The listing builds one solid part. Answer for the finished solid, in the listing's coordinates (mm). A direction names the side the tool comes from. Give positions to 0.01 mm unless a question says otherwise; leave off trailing zeros. Write each loop counter-clockwise with the first axis right and the second up, starting at its lowest first coordinate (ties: lowest second). Pieces come first, ordered by that corner, then holes. Notation, with made-up numbers: (23, 64) - (60, 64) arc R33 ccw to (60, 95) - close; hole circle Ø3 at (59.5, 39). An arc over 180 degrees is marked (long way). Write each question's results on one line, items separated by ' | '. Start each with the question number.
Q1. Section B-B (x = 0) is taken. State how many separate pieces and enclosed holes the cut face has, plus the area to 3 significant figures.
Q2. For faces 4 (the face through (0.364, 0.967, 18.076)), 5 (the face through (-0.28, 10.312, 33.866)), 6 (the face through (-10.325, -1.464, 1.479)), 7 (the face through (0, 13, 2)), 8 (the face through (0, 3, 4)), determine the directions among +Z, -Z, +X, -X, +Y, -Y from which every point of the face is accessible in a straight line to the end or side of a thin tool.
Q3. Section A-A (z = 8) is taken. Determine the outline of the cut face in (x, y), plus the area to 3 significant figures.
Q4. Section C-C (y = 41.5) is taken. Determine the outline of the cut face in (x, z).
Q5. For a pull along Z with two mould halves and no side action, classify faces 1 (the face through (-18.498, 44.726, 45.771)), 2 (the face through (-9.3, 1.5, 3)), 3 (the face through (-28, 14.7, 15.4)) as pulls with the +Z half, pulls with the -Z half, needs draft (parallel to the pull), parting line crosses it, or undercut.
Q6. Find the intervals of material crossed by probe 1 along X at (y, z) = (0.5, 18); probe 2 along Z at (x, y) = (19.5, 25.5); probe 3 along Z at (x, y) = (0.5, 10.5), in increasing order.
Q7. Flat-ended cylindrical pins translate along their axes: pin 1 Ø6 at (x, z) = (-21.5, 15.5) entering from -Y; pin 2 Ø15 at (x, y) = (4, 30) entering from -Z; pin 3 Ø5 at (y, z) = (38.5, 42.5) entering from -X; pin 4 Ø4 at (x, z) = (-19, 15.5) entering from -Y. Find the tip coordinate at first contact, or state that the pin passes through.
```python
from build123d import *

# Parameters (mm, degrees)
SKETCH_1_R          = 1.4999999999999987
EXTRUDE_1_DEPTH     = 4
SKETCH_3_R          = 3.2499999999999996
SKETCH_3_R_2        = 3.249999999999999
CUT_EXTRUDE_1_DEPTH = 1
EXTRUDE_2_DEPTH     = 4
EXTRUDE_3_DEPTH     = 4
EXTRUDE_4_DEPTH     = 52
FILLET_1_R          = 25
FILLET_2_R          = 20
EXTRUDE_6_DEPTH     = 52
FILLET_4_R          = 6
FILLET_5_R          = 2
SKETCH_11_R         = 7.500000000000031
CUT_EXTRUDE_2_DEPTH = 4
FILLET_6_R          = 2


with BuildPart() as part:
    # 草图1 → 凸台-拉伸1 (new body)
    # profile 1 of 3: a face of its own
    with BuildSketch(Plane.XY):
        Polygon((30.00000000000006, 4.99999999999999), (30.000000000000057, -5.0000000000000115), (-29.99999999999994, -5.0000000000000115), (-29.999999999999936, 4.99999999999999), align=None)
        with Locations((9.999999999999996, 5.68e-15)):
            Circle(SKETCH_1_R, mode=Mode.SUBTRACT)
        with Locations((-10.000000000000004, -4.4e-16)):
            Circle(SKETCH_1_R, mode=Mode.SUBTRACT)
    # profile 2 of 3: a face of its own
    with BuildSketch(Plane.XY):
        Polygon((-30.000000000000014, 12.999999999999998), (29.999999999999986, 12.999999999999998), (30.00000000000006, 4.99999999999999), (-29.999999999999936, 4.99999999999999), align=None)
    # profile 3 of 3: a face of its own
    with BuildSketch(Plane.XY):
        Polygon((-29.99999999999994, -5.0000000000000115), (-30.000000000000018, -8.000000000000002), (29.999999999999982, -8.000000000000002), (30.000000000000057, -5.0000000000000115), align=None)
    extrude(amount=EXTRUDE_1_DEPTH)

    # 草图3 → 切除-拉伸1 (cut)
    with BuildSketch(Plane.XY.offset(4)):
        with Locations((-10.000000000000004, -4.6e-16)):
            Circle(SKETCH_3_R)
        with Locations((9.999999999999996, 5.69e-15)):
            Circle(SKETCH_3_R_2)
    extrude(amount=-CUT_EXTRUDE_1_DEPTH, mode=Mode.SUBTRACT)

    # 草图5 → 凸台-拉伸2 (add)
    with BuildSketch(Plane.ZY.offset(29.999999999999936)):
        Polygon((47.25000000000001, 15.99999999999999), (4, -8.000000000000012), (4, 12.999999999999988), (44.25, 18.99999999999999), (44.25, 64.99999999999999), (47.25, 64.99999999999999), align=None)
    extrude(amount=-EXTRUDE_2_DEPTH)

    # 草图6 → 凸台-拉伸3 (add)
    with BuildSketch(Plane(origin=(30.00000000000006, -1.041e-14, 0), x_dir=(0, 0, -1), z_dir=(1, -3.5e-16, 0))):
        Polygon((-44.25, 64.99999999999999), (-47.25, 64.99999999999999), (-47.25000000000001, 15.99999999999999), (-4, -8.00000000000001), (-4, 13.000000000000009), (-44.25, 18.999999999999993), align=None)
    extrude(amount=-EXTRUDE_3_DEPTH)

    # 草图7 → 凸台-拉伸4 (add)
    with BuildSketch(Plane(origin=(-25.999999999999932, 8.47e-15, 0), x_dir=(0, 0, -1), z_dir=(1, -3.3e-16, 0))):
        Polygon((-44.25, 14.335260115606923), (-44.25, 18.999999999999993), (-44.25, 64.99999999999999), (-47.25, 64.99999999999999), (-47.25000000000001, 15.999999999999986), align=None)
    extrude(amount=EXTRUDE_4_DEPTH)

    # 圆角1
    fillet_1_edges = [part.edges().sort_by_distance(p)[0] for p in [
        (-29.999999999999915, 65, 45.75),
        (30.00000000000008, 64.99999999999997, 45.75),
    ]]
    fillet(fillet_1_edges, radius=FILLET_1_R)

    # 圆角2
    fillet_2_edges = [part.edges().sort_by_distance(p)[0] for p in [
        (-27.99999999999993, 19, 44.25),
        (28.000000000000068, 18.999999999999982, 44.25),
    ]]
    fillet(fillet_2_edges, radius=FILLET_2_R)

    # 草图9 → 凸台-拉伸6 (add)
    with BuildSketch(Plane(origin=(-25.999999999999932, 8.47e-15, 0), x_dir=(0, 0, -1), z_dir=(1, -3.3e-16, 0))):
        Polygon((-33.14820415728187, 11.605667405253392), (-34.60384535674384, 8.982480660389633), (-17.11593372431879, -0.7217940026901655), (-17.115933724318786, 2.7091473962102923), align=None)
    extrude(amount=EXTRUDE_6_DEPTH)

    # 圆角4
    fillet_4_edges = [part.edges().sort_by_distance(p)[0] for p in [
        (-25.99999999999993, 10.294074032821522, 33.87602475701286),
        (26.00000000000007, 10.294074032821504, 33.87602475701286),
    ]]
    fillet(fillet_4_edges, radius=FILLET_4_R)

    # 圆角5
    fillet_5_edges = [part.edges().sort_by_distance(p)[0] for p in [
        (6.75e-14, -0.721794002690165, 17.11593372431879),
    ]]
    fillet(fillet_5_edges, radius=FILLET_5_R)

    # 草图11 → 切除-拉伸2 (cut)
    with BuildSketch(Plane.XY.offset(47.25000000000001)):
        with BuildLine():
            ThreePointArc((-20.11504932930021, 46.93210856983418), (-19.24913556906646, 44.8416078260319), (-17.158634825264187, 45.70752158626565))
            ThreePointArc((-17.158634825264187, 45.70752158626565), (-18.024548585497932, 47.79802233006792), (-20.11504932930021, 46.93210856983418))
        make_face()
        with BuildLine():
            ThreePointArc((-4.207521586267032, 24.341365174733916), (-6.298022330069304, 23.475451414500167), (-5.432108569835557, 21.384950670697894))
            ThreePointArc((-5.432108569835557, 21.384950670697894), (-3.341607826033282, 22.250864430931642), (-4.207521586267032, 24.341365174733916))
        make_face()
        with BuildLine():
            ThreePointArc((20.11504932930082, 36.06789143016255), (19.24913556906707, 38.158392173964835), (17.158634825264798, 37.292478413731075))
            ThreePointArc((17.158634825264798, 37.292478413731075), (18.024548585498543, 35.20197766992881), (20.11504932930082, 36.06789143016255))
        make_face()
        with BuildLine():
            ThreePointArc((5.43210856983612, 61.61504932929888), (3.341607826033848, 60.74913556906513), (4.207521586267595, 58.65863482526286))
            ThreePointArc((4.207521586267595, 58.65863482526286), (6.298022330069867, 59.5245485854966), (5.43210856983612, 61.61504932929888))
        make_face()
        with Locations((2.6021e-13, 41.49999999999841)):
            Circle(SKETCH_11_R)
    extrude(amount=-CUT_EXTRUDE_2_DEPTH, mode=Mode.SUBTRACT)

    # 圆角6
    fillet_6_edges = [part.edges().sort_by_distance(p)[0] for p in [
        (7.105e-14, 15.99999999999999, 47.25000000000001),
    ]]
    fillet(fillet_6_edges, radius=FILLET_6_R)


solid = part.part
```
Answers below:
1) separate pieces: 4 | enclosed holes: 0 | area: 243 mm2
2) face 4: -Y | face 5: +Z, +Y | face 6: -Z | face 7: -Z, +X, -X, +Y | face 8: +Y, -Y
3) outline: (-30, -5.78) - (-26, -5.78) - (-26, 13.6) - (-30, 13.6) - close; (26, -5.78) - (30, -5.78) - (30, 13.6) - (26, 13.6) - close | area: 155 mm2
4) outline: (-29.95, 44.25) - (-7.5, 44.25) - (-7.5, 47.25) - (-29.95, 47.25) - close; (7.5, 44.25) - (29.95, 44.25) - (29.95, 47.25) - (7.5, 47.25) - close
5) face 1: needs draft | face 2: undercut | face 3: pulls with the -Z half
6) probe 1: x = -30 to -26, 26 to 30 | probe 2: z = 44.25 to 47.25 | probe 3: z = 0 to 4, 31.16 to 33.76
7) pin 1: stops at y = 0.77 | pin 2: stops at z = 44.25 | pin 3: stops at x = -30 | pin 4: stops at y = 1.5
